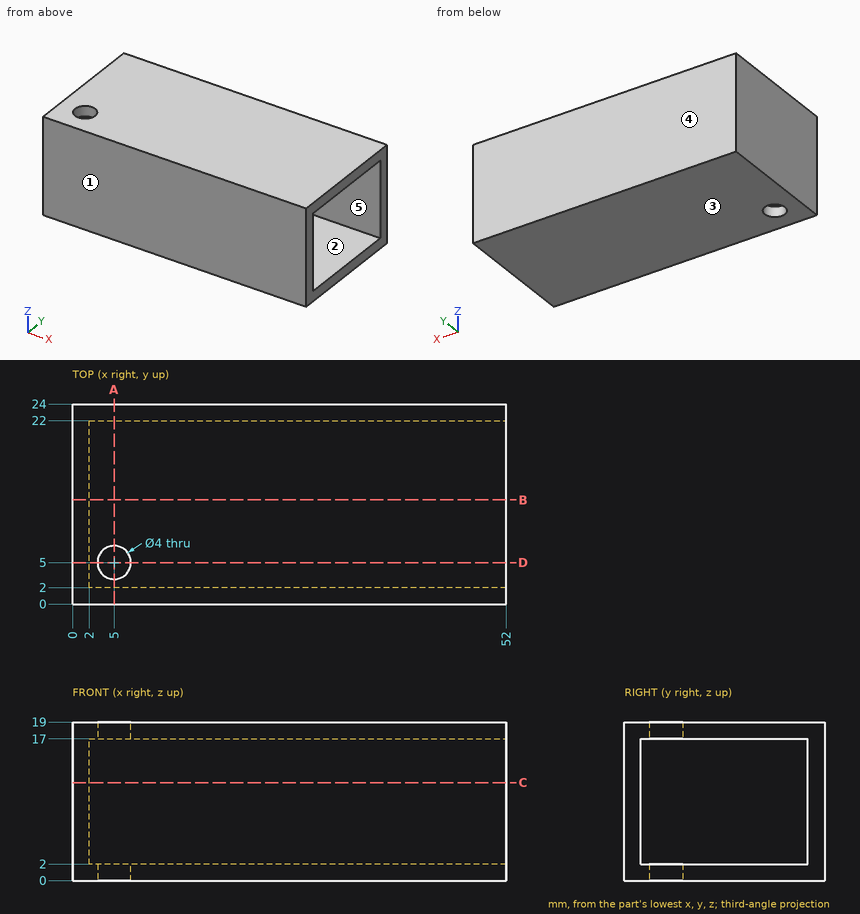
Design review of the part shown in the three views and the two pictorial views. Dimensions are in mm from the part's minimum x, y and z. A direction names the side the tool comes from. Give positions to 0.01 mm unless a question says otherwise; leave off trailing zeros. Loops run counter-clockwise (first coordinate to the right, second up) from the corner with the lowest first, then second, coordinate; pieces in that order, holes last. Notation, with made-up numbers: M -17.75,86 L 30.25,86 A10 ccw 30.25,95 Z; hole C 59,73.5 d8. An arc over 180 degrees is marked long. Put each result on its own line as item: value. Start each with the question number.
(1) Add section A-A, the plane x = 5. Write out the cut boundary in (y, z).
(2) Wall thickness on L1, parallel to Y at x = 25, z = 10.75; L2, parallel to Y at x = 5, z = 1.1; L3, parallel to Z at x = 26, y = 7: over which ranges is each line inside the solid? List them lowest first.
(3) For pin 1 (7.5 mm diameter, centred on y = 11, z = 9, fed in from +X), flat-tipped, find the tip position at first contact; note if it passes through.
(4) Add section B-B, the plane y = 12.5. Write out the cut boundary in (x, z).
(5) Add section C-C, the plane z = 11.75. Write out the cut boundary in (x, y).
(6) The part is to be moulded in two halves that separate along Y. For the marked faces 3, 4 and 5, say which applies: +Y half, -Y half, draft (parallel to the pull), parting line (faces both ways), or undercut.
(7) Machinability: for the marked faces 1 and 2, which of the approach directions +Z, -Z, +X, -X, +Y, -Y give a long, thin tool a straight path to every point of the face, cutting with its end or side? Answer none if there is none.
(8) Add section D-D, the plane y = 5. Write out the cut boundary in (x, z).
Result:
1. outline: M 0,0 L 3,0 L 3,2 L 2,2 L 2,17 L 3,17 L 3,19 L 0,19 Z; M 7,0 L 24,0 L 24,19 L 7,19 L 7,17 L 22,17 L 22,2 L 7,2 Z
2. L1: y = 0 to 2, 22 to 24
2. L2: y = 0 to 3, 7 to 24
2. L3: z = 0 to 2, 17 to 19
3. pin 1: stops at x = 2
4. outline: M 0,0 L 52,0 L 52,2 L 2,2 L 2,17 L 52,17 L 52,19 L 0,19 Z
5. outline: M 0,0 L 52,0 L 52,2 L 2,2 L 2,22 L 52,22 L 52,24 L 0,24 Z
6. face 3: draft
6. face 4: +Y half
6. face 5: undercut
7. face 1: +Z, -Z, +X, -X, -Y
7. face 2: +X
8. outline: M 0,0 L 3,0 L 3,2 L 2,2 L 2,17 L 3,17 L 3,19 L 0,19 Z; M 7,0 L 52,0 L 52,2 L 7,2 Z; M 7,17 L 52,17 L 52,19 L 7,19 Z
